Design review of the part built by this model. Coordinates are the model's own, in mm. Face numbers are marked on the shaded views. Coordinates: 2 decimals unless noted, no trailing zeros. Loops run counter-clockwise (first coordinate to the right, second up) from the corner with the lowest first, then second, coordinate; pieces in that order, holes last. Notation, with made-up numbers: (46, 7.5) -> (65, 7.5) arc R17 cw to (65, 25.5) -> close; hole circle Ø7 at (4.5, -40). An arc over 180 degrees is marked (long way). Use a Markdown table: item, result. Add a question column.
Q1. Clearance check with flat-ended pins moving along their axes: pin 1 Ø5 at (x, y) = (42.5, 0) entering from -Z; pin 2 Ø10 at (x, y) = (9, 54) entering from +Z; pin 3 Ø2 at (x, y) = (20, -49.5) entering from -Z. State where each tip first meets the part, or that it passes through.
Q2. Take a section at B-B on y = 59.5. Write out the cut boundary in (x, z), plus the area to 3 significant figures.
Q3. Draft analysis for pull direction X (two halves, no side actions). For the marked faces 1, 2 and 3, state which applies: pulls with the +X half, pulls with the -X half, needs draft (parallel to the pull), parting line crosses it, or undercut.
Q4. Take a section at A-A on x = 0. Write out the cut boundary in (y, z), plus the area to 3 significant figures.
Q5. Take a section at D-D on y = -50.5. Write out the cut boundary in (x, z), plus the area to 3 significant figures.
Q6. For probe 1 along Z at (x, y) = (0, 46); probe 2 along Z at (x, y) = (0, 38.5), list the stretches that pass through material, from the lowest coordinate up.
Q7. Take a section at C-C on z = 0. Write out the cut boundary in (x, y).
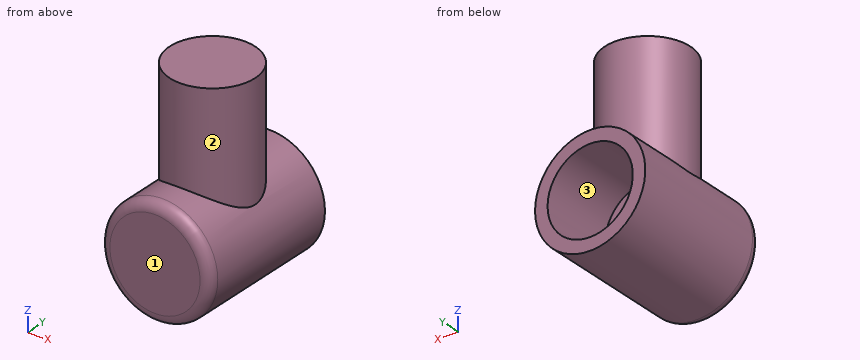
from build123d import *

# Parameters (mm, degrees)
SKETCH1_R           = 55
BOSS_EXTRUDE1_DEPTH = 75
SKETCH2_R           = 42.5
BOSS_EXTRUDE2_DEPTH = 150
FILLET2_R           = 10
SKETCH3_R           = 42.5
CUT_EXTRUDE1_DEPTH  = 110


with BuildPart() as part:
    # Sketch1 → Boss-Extrude1 (new body, symmetric)
    with BuildSketch(Plane(origin=(0, 0, 0), x_dir=(1, 0, 0), z_dir=(0, 1, 0))):
        Circle(SKETCH1_R)
    extrude(amount=BOSS_EXTRUDE1_DEPTH, both=True)

    # Sketch2 → Boss-Extrude2 (add)
    with BuildSketch(Plane.XY):
        Circle(SKETCH2_R)
    extrude(amount=BOSS_EXTRUDE2_DEPTH)

    # Fillet2
    fillet2_edges = [part.edges().sort_by_distance(p)[0] for p in [
        (-55, -75, 0),
    ]]
    fillet(fillet2_edges, radius=FILLET2_R)

    # Sketch3 → Cut-Extrude1 (cut)
    with BuildSketch(Plane(origin=(0, 0, 0), x_dir=(1, 0, 0), z_dir=(0, 1, 0))):
        Circle(SKETCH3_R)
    extrude(amount=CUT_EXTRUDE1_DEPTH, mode=Mode.SUBTRACT)


solid = part.part
Answer list:
| question | item | result |
|---|---|---|
| 1 | pin 1 | z = -37.75 |
| 1 | pin 2 | z = 54.85 |
| 1 | pin 3 | z = -51.61 |
| 2 | outline | circle Ø110 at (0, 0); hole circle Ø85 at (0, 0) |
| 2 | area | 3,830 mm² |
| 3 | face 1 | needs draft |
| 3 | face 2 | parting line crosses it |
| 3 | face 3 | undercut |
| 4 | outline | (-75, -45) arc R10 ccw to (-65, -55) -> (75, -55) -> (75, -42.5) -> (0, -42.5) -> (0, 42.5) -> (75, 42.5) -> (75, 55) -> (42.5, 55) -> (42.5, 150) -> (-42.5, 150) -> (-42.5, 55) -> (-65, 55) arc R10 ccw to (-75, 45) -> close |
| 4 | area | 18,200 mm² |
| 5 | outline | circle Ø110 at (0, 0) |
| 5 | area | 9,500 mm² |
| 6 | probe 1 | -55 to -42.5, 42.5 to 55 |
| 6 | probe 2 | -55 to -42.5, 42.5 to 150 |
| 7 | outline | (-55, -65) arc R10 ccw to (-45, -75) -> (45, -75) arc R10 ccw to (55, -65) -> (55, 75) -> (42.5, 75) -> (42.5, 0) -> (-42.5, 0) -> (-42.5, 75) -> (-55, 75) -> close |
